Here's the drawing with two shaded views (mm, measured from the low corner). I have some questions. A direction names the side the tool comes from. Round coordinates to 2 decimals unless told otherwise and drop trailing zeros. Loops run counter-clockwise (first coordinate to the right, second up) from the corner with the lowest first, then second, coordinate; pieces in that order, holes last. Notation, with made-up numbers: M -27.5,61.25 L -22.5,61.25 A24 cw -22.5,90.25 Z; hole C -12.5,-37.5 d11. An arc over 180 degrees is marked long. Answer as a JSON object with one key per item and string values.
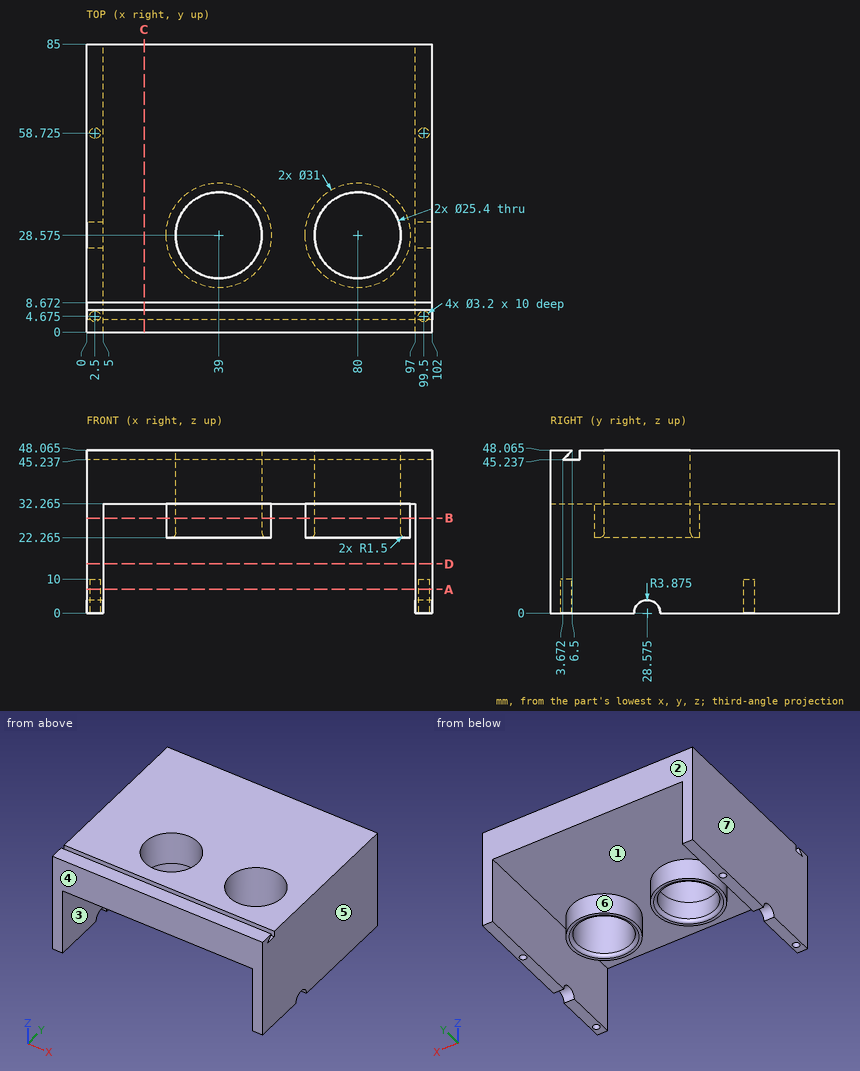
Item 1: I want a section at A-A on z = 7. List the corners of the cut face in (x, y) for me (1 decimal).
Solution:
{"outline": "M 0,0 L 5,0 L 5,85 L 0,85 Z; M 97,0 L 102,0 L 102,85 L 97,85 Z; hole C 2.5,4.7 d3.2; hole C 2.5,58.7 d3.2; hole C 99.5,4.7 d3.2; hole C 99.5,58.7 d3.2"}
Item 2: For P1, Ø25, axis at x = 33, y = 28, coming from the -Z side (3 decimals); P2, Ø2.5, axis at x = 2.5, y = 58.5, coming from the -Z side; P3, Ø5, axis at x = 33.5, y = 23, coming from the +Z side, each with a flat end and sliding along its axis, tell me the tip position at first contact or that it passes through.
Solution:
{"P1": "stops at z = 22.265", "P2": "stops at z = 10", "P3": "passes through"}
Item 3: If I drill on L1, parallel to X at y = 24, z = 4; L2, parallel to Y at x = 99, z = 7 (1 decimal); L3, parallel to Z at x = 32.5, y = 71 (1 decimal), over which ranges is the centre line in solid material (lowest first)? Write a range as from..to.
Solution:
{"L1": "x = 0..5, 97..102", "L2": "y = 0..3.2, 6.2..57.2, 60.2..85", "L3": "z = 32.3..48.1"}
Item 4: We'd pull the mould along X, two halves only. Please class the marked faces 4, 5, 6 and 7: +X half, -X half, draft (parallel to the pull), parting line (faces both ways), or undercut.
Solution:
{"face 4": "draft", "face 5": "+X half", "face 6": "undercut", "face 7": "-X half"}
Item 5: I want a section at D-D on z = 14.5. List the corners of the cut face in (x, y) for me.
Solution:
{"outline": "M 0,0 L 5,0 L 5,85 L 0,85 Z; M 97,0 L 102,0 L 102,85 L 97,85 Z"}
Item 6: I want a section at B-B on z = 28. List the corners of the cut face in (x, y) for me (1 decimal).
Solution:
{"outline": "M 0,0 L 5,0 L 5,85 L 0,85 Z; C 39,28.6 d31; C 80,28.6 d31; M 97,0 L 102,0 L 102,85 L 97,85 Z; hole C 39,28.6 d25.4; hole C 80,28.6 d25.4"}
Item 7: For the marked faces 1, 2 and 3, which set-ups out of +Z, -Z, +X, -X, +Y, -Y let a thin tool reach every point of the face, with its end or its side?
Solution:
{"face 1": "-Z", "face 2": "+Z, -Z, +X, -X, +Y", "face 3": "-Z, +Y, -Y"}
Item 8: I want a section at C-C on x = 17. List the corners of the cut face in (y, z) for me (1 decimal).
Solution:
{"outline": "M 0,32.3 L 85,32.3 L 85,48.1 L 8.7,48.1 L 8.7,45.2 L 3.7,45.2 L 6.5,48.1 L 0,48.1 Z"}
